```python
from build123d import *

# Parameters (mm, degrees)
BOSS_EXTRUDE1_DEPTH = 1
SKETCH2_W           = 1
SKETCH2_H           = 15
BOSS_EXTRUDE2_DEPTH = 3
SKETCH4_R           = 1.190073959
CUT_EXTRUDE1_DEPTH  = 3


with BuildPart() as part:
    # Sketch1 → Boss-Extrude1 (new body)
    with BuildSketch(Plane.XY):
        Polygon((0, 0), (7, 0), (7, 7), (1, 7), (1, 15), (0, 15), align=None)
    extrude(amount=BOSS_EXTRUDE1_DEPTH)

    # Sketch2 → Boss-Extrude2 (add)
    with BuildSketch(Plane(origin=(0, 0, 0), x_dir=(-1, 0, 0), z_dir=(0, 0, -1))):
        with Locations((-0.5, 7.5)):
            Rectangle(SKETCH2_W, SKETCH2_H)
    extrude(amount=BOSS_EXTRUDE2_DEPTH)

    # Sketch4 → Cut-Extrude1 (cut)
    with BuildSketch(Plane.XY.offset(1)):
        with Locations((4, 2.5)):
            Circle(SKETCH4_R)
    extrude(amount=-CUT_EXTRUDE1_DEPTH, mode=Mode.SUBTRACT)


solid = part.part
```
For this review, take the finished solid that the model builds, in its own axes (mm). A direction names the side the tool comes from. Coordinates: 2 decimals unless noted, no trailing zeros. Write each loop counter-clockwise with the first axis right and the second up, starting at its lowest first coordinate (ties: lowest second). Pieces come first, ordered by that corner, then holes. Notation, with made-up numbers: (-25, 14.25) - (1, 14.25) arc R19 ccw to (1, 44.25) - close; hole circle Ø3 at (-24, -34). An arc over 180 degrees is marked (long way). Answer in a Markdown table with one row per item. Add a question column.
Q1. We need section D-D, the plane x = 5. State the section outline as (y, z) points.
Q2. Draft analysis for pull direction X (two halves, no side actions). For faces 1 (the cylindrical face through (3.056, 1.776, 0.507)), 2 (the flat face through (0, 7, -1)), 3 (the flat face through (7, 3.5, 0.5)), 4 (the flat face through (3, 4, 1)), state which applies: +X half, -X half, draft (parallel to the pull), parting line (faces both ways), or undercut.
Q3. For P1, Ø2, axis at y = 7.5, z = -1.5, coming from the +X side; P2, Ø3, axis at x = 5, y = 2, coming from the -Z side; P3, Ø4, axis at x = 4, y = 13, coming from the -Z side, all flat-tipped, find the tip position at first contact; note any pin that passes through.
Q4. We need section B-B, the plane z = 0.4. State the section outline as (x, y) points.
Q5. Tool access review of faces 5 (the flat face through (2.5, 0, 0.2)), 6 (the flat face through (3, 4, 0)), 7 (the flat face through (4, 7, 0.5)): name each direction out of +Z, -Z, +X, -X, +Y, -Y from which nothing blocks a thin tool from reaching the whole face with its end or side.
Q6. We need section A-A, the plane x = 4. State the section outline as (y, z) points, and give its area (3 significant figures).
Q7. We need section C-C, the plane y = 2.5. State the section outline as (x, z) points, and give its area (3 significant figures).
Q8. For probe 1 along Y at (x, z) = (4, 0.7); probe 2 along X at (y, z) = (11.5, -0.1), list the stretches that pass through material, from the lowest coordinate up.
Answer list:
| question | item | result |
|---|---|---|
| 1 | outline | (0, 0) - (1.85, 0) - (1.85, 1) - (0, 1) - close; (3.15, 0) - (7, 0) - (7, 1) - (3.15, 1) - close |
| 2 | face 1 | undercut |
| 2 | face 2 | -X half |
| 2 | face 3 | +X half |
| 2 | face 4 | draft |
| 3 | P1 | stops at x = 1 |
| 3 | P2 | stops at z = 0 |
| 3 | P3 | passes through |
| 4 | outline | (0, 0) - (7, 0) - (7, 7) - (1, 7) - (1, 15) - (0, 15) - close; hole circle Ø2.38 at (4, 2.5) |
| 5 | face 5 | +Z, -Z, +X, -X, -Y |
| 5 | face 6 | -Z, +X, +Y, -Y |
| 5 | face 7 | +Z, -Z, +X, +Y |
| 6 | outline | (0, 0) - (1.31, 0) - (1.31, 1) - (0, 1) - close; (3.69, 0) - (7, 0) - (7, 1) - (3.69, 1) - close |
| 6 | area | 4.62 mm2 |
| 7 | outline | (0, -3) - (1, -3) - (1, 0) - (2.81, 0) - (2.81, 1) - (0, 1) - close; (5.19, 0) - (7, 0) - (7, 1) - (5.19, 1) - close |
| 7 | area | 7.62 mm2 |
| 8 | probe 1 | y = 0 to 1.31, 3.69 to 7 |
| 8 | probe 2 | x = 0 to 1 |
